Part print with two shaded views. Sizes in mm from the minimum x, y, z corner. A direction names the side the tool comes from. Coordinates: 2 decimals unless noted, no trailing zeros. Write each loop counter-clockwise with the first axis right and the second up, starting at its lowest first coordinate (ties: lowest second). Pieces come first, ordered by that corner, then holes.
Q1. Band-saw the part on D-D, the plane x = 1.25. Write the cut outline in (y, z) (3 decimals), plus the area to 3 significant figures.
Q2. Pin check, flat tips, straight feed: P1, Ø3, axis at x = 6.5, z = 2.5, coming from the -Y side; P2, Ø3, axis at y = 9, z = 3, coming from the -X side; P3, Ø1.8, axis at y = 9.5, z = 2.5, coming from the +X side. Stop position of each tip, or through.
Q3. Which spindle directions (+Z, -Z, +X, -X, +Y, -Y) get a long thin tool onto all of the face, cutting with end or side? Do the marked faces 1 and 2. Say none if no direction does.
Q4. Pull direction Z, two halves, no side cores. Call the marked faces 3, 4, 5 and 6: released by +Z, released by -Z, zero draft, split by the parting line, or undercut.
Q5. Band-saw the part on B-B, the plane z = 3. Write the cut outline in (x, y) (1 decimal), plus the area to 3 significant figures.
Q6. Drill centre lines: probe 1 along X at (y, z) = (13.7, 3); probe 2 along Z at (x, y) = (1.15, 3) (3 decimals); probe 3 along Z at (x, y) = (4.92, 14.35). Where is each one in solid material? Low to high.
Q7. Band-saw the part on A-A, the plane y = 3. Write the cut outline in (x, z) (3 decimals), plus the area to 3 significant figures.
Q8. Band-saw the part on C-C, the plane x = 4.92. Write the cut outline in (y, z).
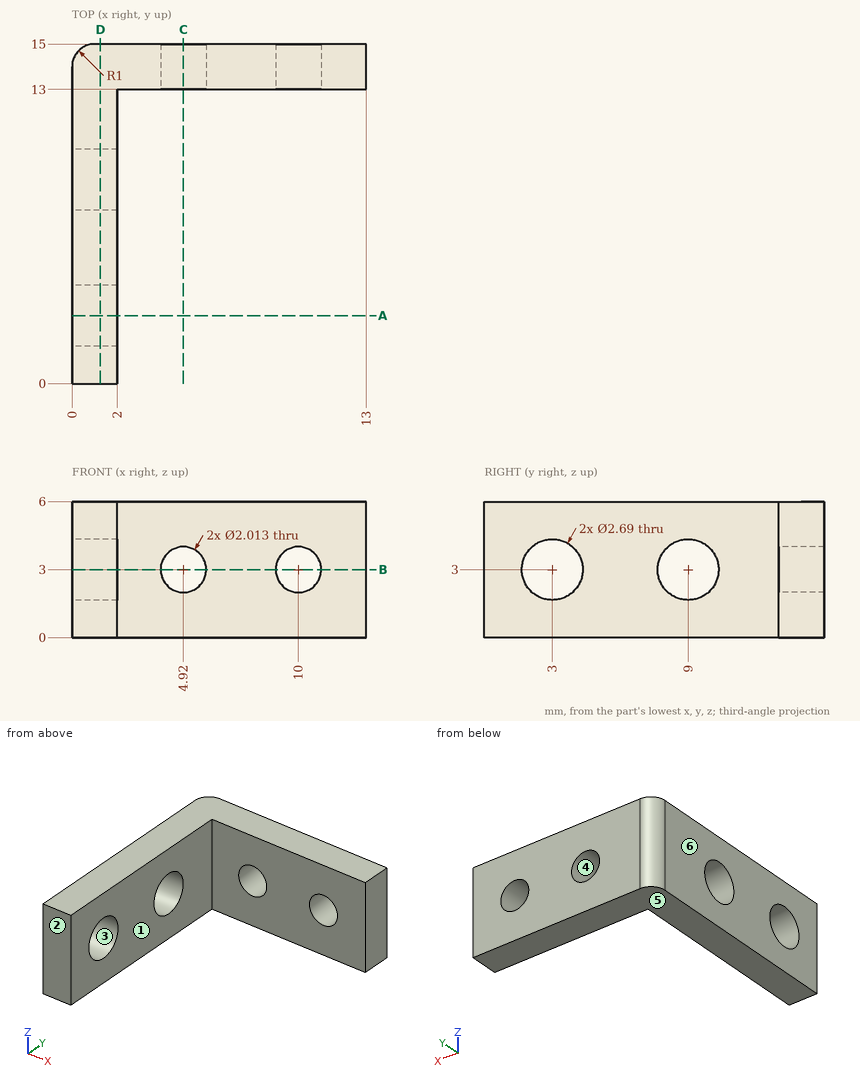
Answer sheet:
1. outline: (0, 0) - (15, 0) - (15, 6) - (0, 6) - close; hole circle Ø2.69 at (3, 3); hole circle Ø2.69 at (9, 3)
1. area: 78.6 mm2
2. P1: stops at y = 13
2. P2: stops at x = 0
2. P3: stops at x = 2
3. face 1: +Z, -Z, +X, -Y
3. face 2: +Z, -Z, +X, -X, -Y
4. face 3: undercut
4. face 4: undercut
4. face 5: released by -Z
4. face 6: zero draft
5. outline: (0, 0) - (2, 0) - (2, 1.7) - (0, 1.7) - close; (0, 4.3) - (2, 4.3) - (2, 7.7) - (0, 7.7) - close; (0, 10.3) - (2, 10.3) - (2, 13) - (3.9, 13) - (3.9, 15) - (1, 15) arc R1 ccw to (0, 14) - close; (5.9, 13) - (9, 13) - (9, 15) - (5.9, 15) - close; (11, 13) - (13, 13) - (13, 15) - (11, 15) - close
5. area: 33.0 mm2
6. probe 1: x = 0 to 3.91, 5.93 to 8.99, 11.01 to 13
6. probe 2: z = 0 to 1.655, 4.345 to 6
6. probe 3: z = 0 to 1.99, 4.01 to 6
7. outline: (0, 0) - (2, 0) - (2, 1.655) - (0, 1.655) - close; (0, 4.345) - (2, 4.345) - (2, 6) - (0, 6) - close
7. area: 6.62 mm2
8. outline: (13, 0) - (15, 0) - (15, 1.99) - (13, 1.99) - close; (13, 4.01) - (15, 4.01) - (15, 6) - (13, 6) - close
